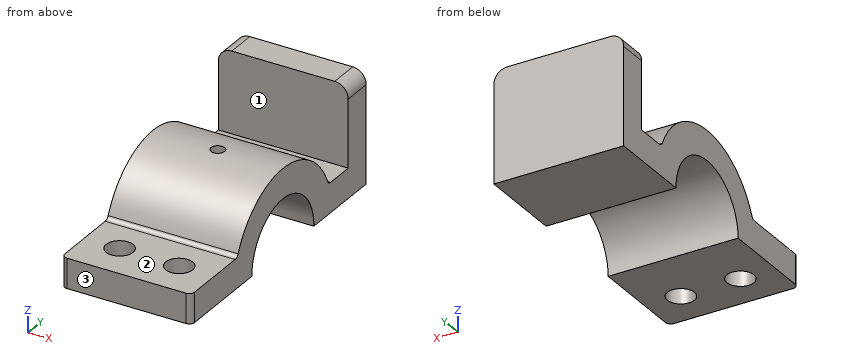
from build123d import *

# Parameters (mm, degrees)
F0_W     = 11
F0_H     = 30
F1_DEPTH = 24
F3_DEPTH = 25
F4_R     = 2.5
F4_R_2   = 5
F5_DEPTH = 41.001
F6_R     = 2
F7_R     = 5
F8_R     = 2


with BuildPart() as f1:
    # F0 (on Right) → F1 (new body, symmetric)
    with BuildSketch(Plane.YZ):
        with BuildLine():
            Line((-56, 0), (-30, 0))
            ThreePointArc((-30, 0), (-29.4730143031, 5.5983415304), (-27.9105714739, 11))
            Line((-27.9105714739, 11), (-56, 11))
            Line((-56, 11), (-56, 0))
        make_face()
        with BuildLine():
            Line((-30, 0), (-19, 0))
            ThreePointArc((-19, 0), (-18.1017503893, 5.7729223833), (-15.4919333848, 11))
            Line((-15.4919333848, 11), (-27.9105714739, 11))
            ThreePointArc((-27.9105714739, 11), (-29.4730143031, 5.5983415304), (-30, 0))
        make_face()
        with BuildLine():
            ThreePointArc((15.4919333848, 11), (18.1017503893, 5.7729223833), (19, 0))
            Line((19, 0), (30, 0))
            ThreePointArc((30, 0), (29.4730143031, 5.5983415304), (27.9105714739, 11))
            Line((27.9105714739, 11), (15.4919333848, 11))
        make_face()
        with BuildLine():
            ThreePointArc((-15.4919333848, 11), (0, 19), (15.4919333848, 11))
            Line((15.4919333848, 11), (27.9105714739, 11))
            ThreePointArc((27.9105714739, 11), (0, 30), (-27.9105714739, 11))
            Line((-27.9105714739, 11), (-15.4919333848, 11))
        make_face()
        with BuildLine():
            ThreePointArc((27.9105714739, 11), (29.4730143031, 5.5983415304), (30, 0))
            Line((30, 0), (51, 0))
            Line((51, 0), (51, 11))
            Line((51, 11), (40, 11))
            Line((40, 11), (27.9105714739, 11))
        make_face()
        with Locations((45.5, 26)):
            Rectangle(F0_W, F0_H)
    extrude(amount=F1_DEPTH, both=True)

    # F2 (on face) → F3 (cut)
    with BuildSketch(Plane(origin=(0, 51, 0), x_dir=(-1, 0, 0), z_dir=(0, 1, 0))):
        with BuildLine():
            ThreePointArc((-6.5, 25), (0, 18.5), (6.5, 25))
            ThreePointArc((6.5, 25), (0, 31.5), (-6.5, 25))
        make_face()
        with BuildLine():
            ThreePointArc((-6.5, 25), (0, 31.5), (6.5, 25))
            Line((6.5, 25), (6.5, 41))
            Line((6.5, 41), (-6.5, 41))
            Line((-6.5, 41), (-6.5, 25))
        make_face()
    extrude(amount=F3_DEPTH, mode=Mode.SUBTRACT)

    # F4 (on Top) → F5 (cut, through all)
    with BuildSketch(Plane.XY):
        Circle(F4_R)
        with Locations((-11, -41.955285737)):
            Circle(F4_R_2)
        with Locations((11, -41.955285737)):
            Circle(F4_R_2)
    extrude(amount=F5_DEPTH, mode=Mode.SUBTRACT)

    # F6
    f6_edges = [f1.edges().sort_by_distance(p)[0] for p in [
        (24, -56, 5.5),
        (-24, -56, 5.5),
    ]]
    fillet(f6_edges, radius=F6_R)

    # F7
    f7_edges = [f1.edges().sort_by_distance(p)[0] for p in [
        (24, 45.5, 41),
        (-24, 45.5, 41),
    ]]
    fillet(f7_edges, radius=F7_R)

    # F8
    f8_edges = [f1.edges().sort_by_distance(p)[0] for p in [
        (0, -27.910571, 11),
        (0, 27.910571, 11),
    ]]
    fillet(f8_edges, radius=F8_R)


solid = f1.part
Work out the finished part from the listing and answer in its coordinate system (mm). Face numbers are marked on the shaded views. A direction names the side the tool comes from. Coordinates: 2 decimals unless noted, no trailing zeros. Loops run counter-clockwise (first coordinate to the right, second up) from the corner with the lowest first, then second, coordinate; pieces in that order, holes last. Notation, with made-up numbers: (16, 76.25) -> (20, 76.25) arc R22 ccw to (20, 94.25) -> close; hole circle Ø6 at (-36.75, 47). An arc over 180 degrees is marked (long way). Write each question's results on one line, items separated by ' | '. Start each with the question number.
1) Find section B-B on z = 3. Determine the outline of the cut face in (x, y), then the cut area to 3 significant figures.
2) For the marked faces 1, 2 and 3, determine the directions among +Z, -Z, +X, -X, +Y, -Y from which every point of the face is accessible in a straight line to the end or side of a thin tool.
3) Consider line 1 along Y through (x, z) = (11, 3.25); line 2 along Y through (x, z) = (-11, 5); line 3 along X through (y, z) = (0, 23). Determine where each line is inside the solid, lowest interval first.
4) Find section A-A on z = 24. Determine the outline of the cut face in (x, y), then the cut area to 3 significant figures.
5) Find section D-D on z = 17. Determine the outline of the cut face in (x, y).
6) Flat-ended cylindrical pins translate along their axes: P1, Ø3, axis at x = -6.5, y = 28.5, coming from the +Z side; P2, Ø4, axis at x = 13, y = 6, coming from the -Z side; P3, Ø15, axis at x = 8.5, z = 20.5, coming from the -Y side. Find the tip coordinate at first contact, or state that the pin passes through.
7) Find section C-C on x = 11. Determine the outline of the cut face in (y, z).
Response values:
1) outline: (-24, -54) arc R2 ccw to (-22, -56) -> (22, -56) arc R2 ccw to (24, -54) -> (24, -18.76) -> (-24, -18.76) -> close; (-24, 18.76) -> (24, 18.76) -> (24, 51) -> (-24, 51) -> close; hole circle Ø10 at (-11, -41.96); hole circle Ø10 at (11, -41.96) | area: 3,180 mm^2
2) face 1: +Z, +X, -X | face 2: +Z, +X, -X, -Y | face 3: +Z, -Z, +X, -X, -Y
3) line 1: y = -56 to -46.96, -36.96 to -18.72, 18.72 to 51 | line 2: y = -56 to -46.96, -36.96 to -18.33, 18.33 to 51 | line 3: x = -24 to -2.5, 2.5 to 24
4) outline: (-24, -18) -> (24, -18) -> (24, 18) -> (-24, 18) -> close; (-24, 40) -> (24, 40) -> (24, 51) -> (-24, 51) -> close; hole circle Ø5 at (0, 0) | area: 2,240 mm^2
5) outline: (-24, -24.72) -> (24, -24.72) -> (24, -8.49) -> (-24, -8.49) -> close; (-24, 8.49) -> (24, 8.49) -> (24, 24.72) -> (-24, 24.72) -> close; (-24, 40) -> (24, 40) -> (24, 51) -> (-24, 51) -> close
6) P1: stops at z = 13.08 | P2: stops at z = 17.23 | P3: stops at y = -27.04
7) outline: (-56, 0) -> (-46.96, 0) -> (-46.96, 11) -> (-56, 11) -> close; (-36.96, 0) -> (-19, 0) arc R19 cw to (19, 0) -> (51, 0) -> (51, 41) -> (40, 41) -> (40, 11) -> (29.24, 11) arc R2 cw to (27.41, 12.19) arc R30 ccw to (-27.41, 12.19) arc R2 cw to (-29.24, 11) -> (-36.96, 11) -> close
